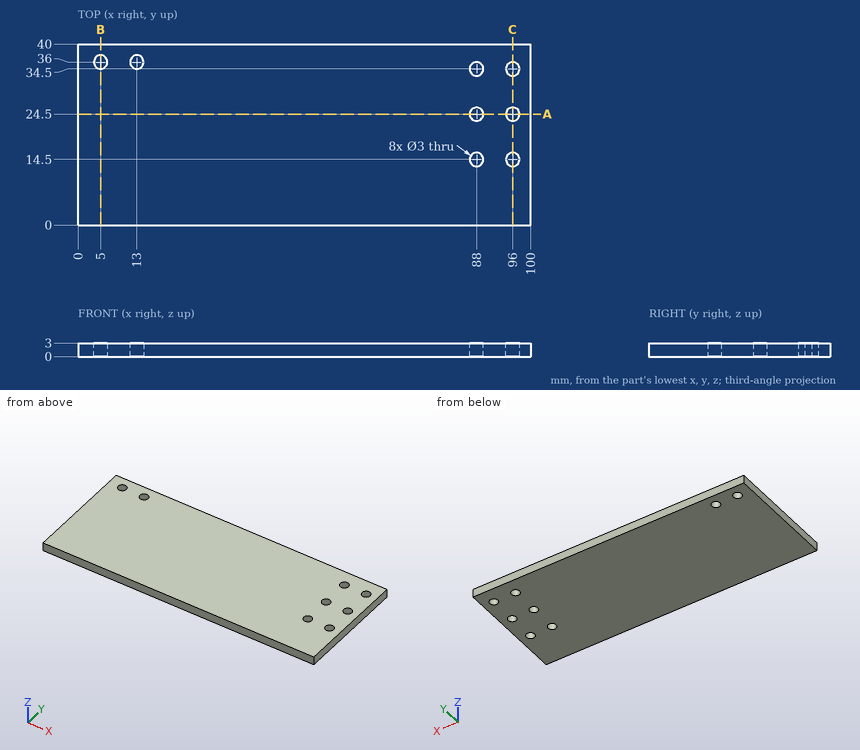
Input: dimensioned drawing with shaded views. Units: mm. Origin: part minimum x, y, z. Coordinates: 2 decimals unless noted, no trailing zeros. Loops run counter-clockwise (first coordinate to the right, second up) from the corner with the lowest first, then second, coordinate; pieces in that order, holes last. Notation, with made-up numbers: M 33,-3 L 89,-3 A17 ccw 89,3 Z; hole C 65,57.25 d4. An arc over 180 degrees is marked long. Put each result on its own line as item: value.
(1) Material intervals for probe 1 along X at (y, z) = (14.5, 1.5); probe 2 along Y at (x, z) = (88, 1.5); probe 3 along X at (y, z) = (15, 2.4), sorted ascending.
Answer sheet:
probe 1: x = 0 to 86.5, 89.5 to 94.5, 97.5 to 100
probe 2: y = 0 to 13, 16 to 23, 26 to 33, 36 to 40
probe 3: x = 0 to 86.59, 89.41 to 94.59, 97.41 to 100
(2) First-contact query: pin 1 (5 mm diameter, centred on x = 88, y = 14.5, fed in from +Z). Flat tip, straight axial feed; report the tip coordinate or a pass-through.
Answer sheet:
pin 1: stops at z = 3
(3) Cut plane C-C on x = 96. Return the cut outline in (y, z).
Answer sheet:
outline: M 0,0 L 13,0 L 13,3 L 0,3 Z; M 16,0 L 23,0 L 23,3 L 16,3 Z; M 26,0 L 33,0 L 33,3 L 26,3 Z; M 36,0 L 40,0 L 40,3 L 36,3 Z
(4) Cut plane B-B on x = 5. Return the cut outline in (y, z).
Answer sheet:
outline: M 0,0 L 34.5,0 L 34.5,3 L 0,3 Z; M 37.5,0 L 40,0 L 40,3 L 37.5,3 Z
(5) Cut plane A-A on y = 24.5. Return the cut outline in (x, z), then the cut area to 3 significant figures.
Answer sheet:
outline: M 0,0 L 86.5,0 L 86.5,3 L 0,3 Z; M 89.5,0 L 94.5,0 L 94.5,3 L 89.5,3 Z; M 97.5,0 L 100,0 L 100,3 L 97.5,3 Z
area: 282 mm^2
